Can you work these out from the model? Positions are in its coordinate system, mm. A direction names the side the tool comes from. Coordinates: 2 decimals unless noted, no trailing zeros. Order: outer loops, then holes, each group sorted by start corner. A loop starts at its lowest first (then second) coordinate and runs counter-clockwise, first axis right, second up. Notation, with made-up numbers: (-28, -27.5) -> (12, -27.5) arc R12 ccw to (12, -14.5) -> close; hole circle Ø10 at (59.5, 71). An arc over 180 degrees is marked (long way). Return JSON: item names as keys, results as strings. Group by question number.
1) If we section it at B-B, the plane z = 0: Please give me the cut outline in (x, y), then the cut area to 3 significant figures.
2) If we section it at C-C, the plane y = 15: Please give me the cut outline in (x, z), then the cut area to 3 significant figures.
3) For faces 1 (the flat face through (-6, 0, 0)), 2 (the cylindrical face through (-3, -3, 0)), 3 (the cylindrical face through (33.958, -0.487, 15.954)), which set-ups out of +Z, -Z, +X, -X, +Y, -Y let a thin tool reach every point of the face, with its end or its side?
4) Thinking about a two-plate mould opening in Z: for faces 4 (the cylindrical face through (44, -3, 0)), 5 (the flat face through (52, 0, 0)), 6 (the conical face through (30.195, 0.012, 17.781)), which applies, +Z half, -Z half, draft (parallel to the pull), parting line (faces both ways), or undercut?
5) If we section it at D-D, the plane x = 8: Please give me the cut outline in (y, z), then the cut area to 3 significant figures.
6) If we section it at A-A, the plane x = 32: Please give me the cut outline in (y, z), then the cut area to 3 significant figures.
7) If I drill on probe 1 along Z at (x, y) = (33.8, 0); probe 2 along X at (y, z) = (-5, -4); probe 3 along Y at (x, z) = (35, -17), over which ranges is the centre line in solid material (lowest first)? Write a range as from..to.
8) For pin 1 (2 mm diameter, centred on x = 36.5, z = 5, fed in from +Y); pin 2 (12 mm diameter, centred on x = 28, y = 1.5, fed in from +Z); pin 3 (5 mm diameter, centred on x = 9.5, z = -14.5, fed in from -Y), each with a flat end and sliding along its axis, tell me the tip position at first contact or that it passes through.
Autodesk Inventor part; units mm, degrees
ref_plane "YZ Plane" through (0, 0, 0) normal (1, 0, 0) x (0, 1, 0)
ref_plane "XZ Plane" through (0, 0, 0) normal (0, 1, 0) x (-1, 0, 0)
ref_plane "XY Plane" through (0, 0, 0) normal (0, 0, 1) x (1, 0, 0)
sketch "Skizze1" plane through (0, 0, 0) normal (0, 0, 1) x (1, 0, 0)
  line L0 (0, 30) -> (0, -5)
  line L1 (-17.6, 0) -> (63.6, 0)
  line L2 (-6, 0) -> (-6, 3)
  line L3 (-6, 3) -> (0, 3)
  line L4 (0, 3) -> (0, 25)
  line L5 (0, 25) -> (37, 25)
  line L6 (37, 25) -> (37, 3)
  line L7 (37, 3) -> (52, 3)
  line L8 (52, 3) -> (52, 0)
  point P0 (0, 0)
  dimension "d0" = 15
  dimension "d2" = 37
  dimension "d3" = 58
  dimension "d4" = 25
  dimension "d5" = 3
  dimension "d6" = 3
revolve "Umdrehung1" add sketch "Skizze1" angle 360 about axis through (0, 0, 0) along (1, 0, 0)
sketch "Skizze2" plane through (37, 0, 0) normal (1, 0, 0) x (0, 0, -1)
  circle A0 centre (0, 0) radius 3
  point P0 (-17.5, 0)
  point P1 (17.5, 0)
  dimension "d8" = 35
  dimension "d9" = 17.5
hole "Bohrung1" at (37, 0, 17.5) at (37, 0, -17.5) direction (-1, 0, 0) diameter 3.242 depth 6 tip angle 118
chamfer "Fase1" distance 0.5 angle 45 2 edges at (52, -3, 0) (-6, -3, 0)
equation "\"d6\" = d5"
properties part number "Motor50" material "Steel"
Result sheet:
{
 "1": {"outline": "(-6, -2.5) -> (-5.5, -3) -> (0, -3) -> (0, -25) -> (37, -25) -> (37, -3) -> (51.5, -3) -> (52, -2.5) -> (52, 2.5) -> (51.5, 3) -> (37, 3) -> (37, 25) -> (0, 25) -> (0, 3) -> (-5.5, 3) -> (-6, 2.5) -> close", "area": "1,980 mm2"},
 "2": {"outline": "(0, -20) -> (37, -20) -> (37, 20) -> (0, 20) -> close", "area": "1,480 mm2"},
 "3": {"face 1": "+Z, -Z, -X, +Y, -Y", "face 2": "-X", "face 3": "+X"},
 "4": {"face 4": "parting line", "face 5": "draft", "face 6": "undercut"},
 "5": {"outline": "circle Ø50 at (0, 0)", "area": "1,960 mm2"},
 "6": {"outline": "circle Ø50 at (0, 0); hole circle Ø3.24 at (0, -17.5); hole circle Ø3.24 at (0, 17.5)", "area": "1,950 mm2"},
 "7": {"probe 1": "z = -25..-19.12, -15.88..15.88, 19.12..25", "probe 2": "x = 0..37", "probe 3": "y = -18.33..-1.54, 1.54..18.33"},
 "8": {"pin 1": "stops at y = 24.68", "pin 2": "stops at z = 25", "pin 3": "stops at y = -21.93"}
}
